```python
from build123d import *

# Parameters (mm, degrees)
F1_DEPTH = 127
F3_DEPTH = 241.3


with BuildPart() as f1:
    # F0 (on Front) → F1 (new body)
    with BuildSketch(Plane.XZ):
        Polygon((155.0226134762, 76.1641544679), (-86.2773865238, 76.1641544679), (-60.8773865238, -112.634918623), (129.6226134762, -112.634918623), align=None)
    extrude(amount=-F1_DEPTH)

    # F2 (on face) → F3 (cut)
    with BuildSketch(Plane(origin=(142.2021087352, 0, -19.131097959), x_dir=(0, 1, 0), z_dir=(0.9910712498, 0, -0.1333333333))):
        Polygon((34.5675349236, -94.3462144431), (0, 96.1537855569), (0, -94.3462144431), align=None)
    extrude(amount=-F3_DEPTH, mode=Mode.SUBTRACT)


solid = f1.part
```
Can you work these out from the model? Positions are in its coordinate system, mm. Give positions to 0.01 mm unless a question says otherwise; leave off trailing zeros. Order: outer loops, then holes, each group sorted by start corner. A loop starts at its lowest first (then second) coordinate and runs counter-clockwise, first axis right, second up. Notation, with made-up numbers: (59.5, 79.25) - (97.5, 79.25) arc R19 cw to (97.5, 85.25) - close; hole circle Ø2 at (73.5, -36.75). An arc over 180 degrees is marked (long way). Use a Markdown table: item, result. Add a question column.
Q1. If we section it at C-C on y = 118: Write out the boundary of the cut face in (x, z), plus the area to 3 significant figures.
Q2. If we section it at A-A on y = 30: Write out the boundary of the cut face in (x, z).
Q3. If we mould it in two halves opening along Z, with no side actions, what happens to faces 1 (the flat face through (33.975, 17.042, -99.767)), 2 (the flat face through (33, 63, -112.635)), 3 (the flat face through (36, 63, 76.164)), 4 (the flat face through (33, 127, -17))? For each: released by +Z, released by -Z, zero draft, split by the parting line, or undercut.
Q4. Please list where these lines run through material, in increasing order: line 1 along Y through (x, z) = (92, -74); line 2 along X through (y, z) = (68.5, -99); line 3 along X through (y, z) = (69, 46.5).
Q5. I'm going to push flat-ended pins straight in: pin 1 (4 mm diameter, centred on y = 94.5, z = -33, fed in from -X); pin 2 (5 mm diameter, centred on y = 102.5, z = 9.5, fed in from -X); pin 3 (1 mm diameter, centred on y = 30.5, z = 23, fed in from -X). Where does each tip first touch, or does it pass through?
Q6. If we section it at B-B on x = 68.5: Write out the boundary of the cut face in (y, z).
Q7. If we section it at D-D on z = 4: Write out the boundary of the cut face in (x, y).
Answers follow:
| question | item | result |
|---|---|---|
| 1 | outline | (-86.28, 76.16) - (-60.88, -112.63) - (129.62, -112.63) - (155.02, 76.16) - close |
| 1 | area | 40,800 mm^2 |
| 2 | outline | (-86.28, 76.16) - (-67.87, -60.67) - (132.98, -87.69) - (155.02, 76.16) - close; (-64.39, -86.53) - (-60.88, -112.63) - (129.62, -112.63) - close |
| 3 | face 1 | undercut |
| 3 | face 2 | released by -Z |
| 3 | face 3 | released by +Z |
| 3 | face 4 | zero draft |
| 4 | line 1 | y = 28.53 to 127 |
| 4 | line 2 | x = -62.71 to 131.46 |
| 4 | line 3 | x = -82.29 to 151.03 |
| 5 | pin 1 | stops at x = -71.86 |
| 5 | pin 2 | stops at x = -77.65 |
| 5 | pin 3 | stops at x = -79.19 |
| 6 | outline | (0, -112.63) - (127, -112.63) - (127, 76.16) - (2.09, 76.16) - (34.57, -104.41) - (0, -104.41) - close |
| 7 | outline | (-76.57, 18.58) - (145.31, 13.21) - (145.31, 127) - (-76.57, 127) - close |
